Can you work these out from the model? Positions are in its coordinate system, mm. Face numbers are marked on the shaded views. A direction names the side the tool comes from. Give positions to 0.01 mm unless a question says otherwise; leave off trailing zeros. Order: outer loops, then holes, each group sorted by start corner. A loop starts at its lowest first (then second) coordinate and runs counter-clockwise, first axis right, second up.
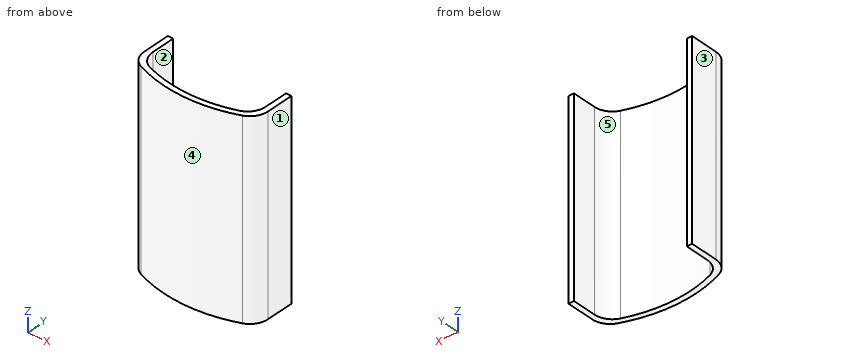
```python
from build123d import *

# Parameters (mm, degrees)
BOSS_EXTRUDE1_DEPTH = 26.9875


with BuildPart() as part:
    # Sketch3 → Boss-Extrude1 (new body)
    with BuildSketch(Plane.XY):
        with BuildLine():
            Line((7.9375, 5.04103367), (7.9375, 1.680064545))
            ThreePointArc((7.9375, 1.680064545), (7.47924218, 0.224746884), (6.269823232, -0.705444243))
            ThreePointArc((6.269823232, -0.705444243), (0, -1.815849828), (-6.269823232, -0.705444243))
            ThreePointArc((-6.269823232, -0.705444243), (-7.47924218, 0.224746884), (-7.9375, 1.680064545))
            Line((-7.9375, 1.680064545), (-7.9375, 5.04103367))
            Line((-7.9375, 5.04103367), (-8.6995, 5.04103367))
            Line((-8.6995, 5.04103367), (-8.6995, 1.15664138))
            ThreePointArc((-8.6995, 1.15664138), (-8.264634287, -0.26462905), (-7.108941233, -1.199236661))
            ThreePointArc((-7.108941233, -1.199236661), (0, -2.577849828), (7.108941233, -1.199236661))
            ThreePointArc((7.108941233, -1.199236661), (8.264634287, -0.26462905), (8.6995, 1.15664138))
            Line((8.6995, 1.15664138), (8.6995, 5.04103367))
            Line((8.6995, 5.04103367), (7.9375, 5.04103367))
        make_face()
    extrude(amount=BOSS_EXTRUDE1_DEPTH)


solid = part.part
```
1) Suppose I cut it at D-D (x = 1.75). Please give me the cut outline in (y, z).
2) We'd pull the mould along X, two halves only. Please class the marked faces 1, 2 and 3: +X half, -X half, draft (parallel to the pull), parting line (faces both ways), or undercut.
3) I'm going to push flat-ended pins straight in: pin 1 Ø5 at (x, z) = (-2.5, 15.5) entering from +Y; pin 2 Ø2 at (x, z) = (-5, 5) entering from -Y; pin 3 Ø1 at (x, z) = (-3.5, 7.5) entering from +Y. Where does each tip first touch, or does it pass through?
4) If I drill on line 1 (X direction, y = 2.25, z = 21.75); line 2 (X direction, y = 0.5, z = 10.5); line 3 (Y direction, x = 7.5, z = 11.5), over which ranges is the centre line in solid material (lowest first)?
5) Suppose I cut it at C-C (y = 0.25). Please give me the cut outline in (x, z).
6) Suppose I cut it at B-B (z = 12). Please give me the cut outline in (x, y), and give its area (3 significant figures).
7) Suppose I cut it at A-A (y = 2.5). Please give me the cut outline in (x, z), and give its area (3 significant figures).
8) Which directions (+Z, -Z, +X, -X, +Y, -Y) give clear straight access to the entire face, cutting with the end or side of a thin tool? Please do the marked faces 4 and 5.
Results:
1. outline: (-2.5, 0) - (-1.73, 0) - (-1.73, 26.99) - (-2.5, 26.99) - close
2. face 1: +X half
2. face 2: undercut
2. face 3: -X half
3. pin 1: stops at y = -1.12
3. pin 2: stops at y = -2.15
3. pin 3: stops at y = -1.37
4. line 1: x = -8.7 to -7.94, 7.94 to 8.7
4. line 2: x = -8.61 to -7.65, 7.65 to 8.61
4. line 3: y = -1 to 0.25
5. outline: (-8.53, 0) - (-7.5, 0) - (-7.5, 26.99) - (-8.53, 26.99) - close; (7.5, 0) - (8.53, 0) - (8.53, 26.99) - (7.5, 26.99) - close
6. outline: (-8.7, 1.16) arc R2.54 ccw to (-7.11, -1.2) arc R19.02 ccw to (7.11, -1.2) arc R2.54 ccw to (8.7, 1.16) - (8.7, 5.04) - (7.94, 5.04) - (7.94, 1.68) arc R2.54 cw to (6.27, -0.71) arc R18.26 cw to (-6.27, -0.71) arc R2.54 cw to (-7.94, 1.68) - (-7.94, 5.04) - (-8.7, 5.04) - close
6. area: 21.3 mm2
7. outline: (-8.7, 0) - (-7.94, 0) - (-7.94, 26.99) - (-8.7, 26.99) - close; (7.94, 0) - (8.7, 0) - (8.7, 26.99) - (7.94, 26.99) - close
7. area: 41.1 mm2
8. face 4: +Z, -Z, -Y
8. face 5: +Z, -Z, +Y
